Geometry: final body of the model. Coordinates: model frame, mm. A direction names the side the tool comes from. Coordinates: 2 decimals unless noted, no trailing zeros. Write each loop counter-clockwise with the first axis right and the second up, starting at its lowest first coordinate (ties: lowest second). Pieces come first, ordered by that corner, then holes. Notation, with made-up numbers: M 58,62.5 L 74,62.5 A33 cw 74,91.5 Z; hole C -17,-18.5 d1. An arc over 180 degrees is marked long. Write item = value, one per line. Start each with the question number.
Item 1: Section C-C on x = 16. Output: boundary loops of the cut face in (y, z).
Item 2: Ray query, L1, parallel to X at y = 70, z = 1.55; L2, parallel to X at y = 36.5, z = 5.7; L3, parallel to Y at x = 103.5, z = 1.35. Return the intervals inside material, ascending. Write a range as [from, to].
Item 3: Section A-A on y = 85.5. Output: boundary loops of the cut face in (x, z).
Item 4: Section B-B on y = -11.5. Output: boundary loops of the cut face in (x, z).
Item 5: Reachability of faces 4 (the flat face through (-4, 10, 6)), 5 (the cylindrical face through (-202.638, -16.025, 2.958)), 6 (the flat face through (-250.45, 74.27, 2.96)) from +Z, -Z, +X, -X, +Y, -Y: full face, straight path, thin tool, end or side. Return the list, or none.
Item 6: Pull-direction query (Y, two-part tool) for faces 1 (the cylindrical face through (-299.994, 0.769, 2.958)), 2 (the cylindrical face through (-217.907, 99.341, 2.958)), 3 (the cylindrical face through (202.495, -15.598, 2.958)); classes: +Y half, -Y half, draft (parallel to the pull), parting line (faces both ways), or undercut.
Item 7: First-contact query: pin 1 Ø2 at (y, z) = (58, 1) entering from -X; pin 2 Ø3 at (x, z) = (166.5, 2.5) entering from +Y; pin 3 Ø1.8 at (x, z) = (64, 2) entering from +Y. Flat tips, straight axial feed; report the tip coordinate or a pass-through.
Item 8: Section D-D on x = 169.5. Output: boundary loops of the cut face in (y, z), plus the area to 3 significant figures.
from build123d import *
from OCP.BRepFilletAPI import BRepFilletAPI_MakeFillet

# Parameters (mm, degrees)
RESSALTO_EXTRUS_O2_DEPTH = 6
FILETE2_R1               = 2
FILETE2_R2               = 0.4
FILETE3_R                = 0.4
FILETE4_R                = 2


with BuildPart() as part:
    # Esbo_o1 → Ressalto-extrus_o2 (new body)
    with BuildSketch(Plane.XY):
        with BuildLine():
            Line((-199.999999999, 0), (199.999999999, 0))
            ThreePointArc((199.999999999, 0), (202.565835097, -15.811388301), (209.999999999, -30))
            Line((209.999999999, -30), (289.999999999, -30))
            ThreePointArc((289.999999999, -30), (299.999014124, 0.31398499), (289.62007067, 30.5))
            ThreePointArc((289.62007067, 30.5), (297.818976076, 75.60635228), (265.815415017, 108.432822474))
            Line((265.815415017, 108.432822474), (246.403986634, 35.988385502))
            ThreePointArc((246.403986634, 35.988385502), (242.72975202, 33.867065158), (240.608431676, 37.541299773))
            Line((240.608431676, 37.541299773), (260.019860059, 109.985736744))
            ThreePointArc((260.019860059, 109.985736744), (218.38507475, 99.736242739), (199.999999999, 61))
            Line((199.999999999, 61), (140, 61))
            Line((140, 61), (150.784643454, 58.387579086))
            Line((150.784643454, 58.387579086), (139.047219324, 52.742194858))
            Line((139.047219324, 52.742194858), (160.085396074, 40.245061921))
            Line((160.085396074, 40.245061921), (137.597498913, 43.437533109))
            Line((137.597498913, 43.437533109), (153.154101004, 34.194272541))
            Line((153.154101004, 34.194272541), (138.26257587, 30.30469508))
            Line((138.26257587, 30.30469508), (144.152507453, 26))
            Line((144.152507453, 26), (149.999999999, 26))
            ThreePointArc((149.999999999, 26), (152.999999999, 23), (149.999999999, 20))
            Line((149.999999999, 20), (-149.999999999, 20))
            ThreePointArc((-149.999999999, 20), (-152.999999999, 23), (-149.999999999, 26))
            Line((-149.999999999, 26), (-144.152507453, 26))
            Line((-144.152507453, 26), (-138.26257587, 30.30469508))
            Line((-138.26257587, 30.30469508), (-153.154101004, 34.194272541))
            Line((-153.154101004, 34.194272541), (-137.597498913, 43.437533109))
            Line((-137.597498913, 43.437533109), (-160.085396074, 40.245061921))
            Line((-160.085396074, 40.245061921), (-139.047219324, 52.742194858))
            Line((-139.047219324, 52.742194858), (-150.784643454, 58.387579086))
            Line((-150.784643454, 58.387579086), (-140, 61))
            Line((-140, 61), (-199.999999999, 61))
            ThreePointArc((-199.999999999, 61), (-218.38507475, 99.736242739), (-260.019860059, 109.985736744))
            Line((-260.019860059, 109.985736744), (-240.608431676, 37.541299773))
            ThreePointArc((-240.608431676, 37.541299773), (-242.72975202, 33.867065158), (-246.403986634, 35.988385502))
            Line((-246.403986634, 35.988385502), (-265.815415017, 108.432822474))
            ThreePointArc((-265.815415017, 108.432822474), (-297.818976076, 75.60635228), (-289.62007067, 30.5))
            ThreePointArc((-289.62007067, 30.5), (-299.999014124, 0.31398499), (-289.999999999, -30))
            Line((-289.999999999, -30), (-209.999999999, -30))
            ThreePointArc((-209.999999999, -30), (-202.565835097, -15.811388301), (-199.999999999, 0))
        make_face()
    extrude(amount=RESSALTO_EXTRUS_O2_DEPTH)

    # Filete2: one fillet with a radius per group of edges: ONE call of the kernel's fillet builder (fillet() takes one radius for all edges)
    filete2_edges_1 = [part.edges().sort_by_distance(p)[0] for p in [
        (139.047219324, 52.742194858, 3),
        (137.597498913, 43.437533109, 3),
        (138.26257587, 30.30469508, 3),
    ]]
    filete2_edges_2 = [part.edges().sort_by_distance(p)[0] for p in [
        (140, 61, 3),
    ]]
    filete2 = BRepFilletAPI_MakeFillet(part.part.solid().wrapped)
    for e in filete2_edges_1:
        filete2.Add(FILETE2_R1, e.wrapped)
    for e in filete2_edges_2:
        filete2.Add(FILETE2_R2, e.wrapped)
    add(Compound.cast(filete2.Shape()), mode=Mode.REPLACE)

    # Filete3
    filete3_edges = [part.edges().sort_by_distance(p)[0] for p in [
        (-140, 61, 3),
    ]]
    fillet(filete3_edges, radius=FILETE3_R)

    # Filete4
    filete4_edges = [part.edges().sort_by_distance(p)[0] for p in [
        (-139.047219324, 52.742194858, 3),
        (-137.597498913, 43.437533109, 3),
        (-138.26257587, 30.30469508, 3),
    ]]
    fillet(filete4_edges, radius=FILETE4_R)


solid = part.part
Responses:
q1.outline = M 0,0 L 20,0 L 20,6 L 0,6 Z
q2.L1 = [-299.18, -255.52], [-249.31, -200.82], [200.82, 249.31], [255.52, 299.18]
q2.L2 = [-293.59, -246.54], [-240.52, -149.27], [149.27, 240.52], [246.54, 293.59]
q2.L3 = [0, 20]
q3.outline = M -293.59,0 L -259.67,0 L -259.67,6 L -293.59,6 Z; M -253.46,0 L -206.41,0 L -206.41,6 L -253.46,6 Z; M 206.41,0 L 253.46,0 L 253.46,6 L 206.41,6 Z; M 259.67,0 L 293.59,0 L 293.59,6 L 259.67,6 Z
q4.outline = M -298.66,0 L -201.34,0 L -201.34,6 L -298.66,6 Z; M 201.34,0 L 298.66,0 L 298.66,6 L 201.34,6 Z
q5.face_4 = +Z, +X, -X, +Y, -Y
q5.face_5 = +Z, -Z, -Y
q5.face_6 = +Z, -Z
q6.face_1 = undercut
q6.face_2 = +Y half
q6.face_3 = -Y half
q7.pin_1 = -299.96
q7.pin_2 = 61
q7.pin_3 = 20
q8.outline = M 0,0 L 61,0 L 61,6 L 0,6 Z
q8.area = 366 mm²
